Here's how the part is built. I have some questions about the finished solid (model axes, mm). A direction names the side the tool comes from. Give positions to 0.01 mm unless a question says otherwise; leave off trailing zeros. Write each loop counter-clockwise with the first axis right and the second up, starting at its lowest first coordinate (ties: lowest second). Pieces come first, ordered by that corner, then holes. Notation, with made-up numbers: M 78.25,42.5 L 128.25,42.5 A35 cw 128.25,79.5 Z; hole C 22,77 d1. An arc over 180 degrees is marked long. Use one line per item in the form item = value. Start each with the question number.
Autodesk Inventor part; units mm, degrees
ref_plane "YZ Plane" through (0, 0, 0) normal (1, 0, 0) x (0, 1, 0)
ref_plane "XZ Plane" through (0, 0, 0) normal (0, 1, 0) x (-1, 0, 0)
ref_plane "XY Plane" through (0, 0, 0) normal (0, 0, 1) x (1, 0, 0)
sketch "Sketch1" plane through (0, 0, 0) normal (0, 0, 1) x (1, 0, 0)
  line L0 (0, 0) -> (0, -635)
  line L1 (0, 0) -> (572.8366, -208.4955)
  line L2 (0, 0) -> (609.6, 0) construction
  line L3 (572.8366, -208.4955) -> (572.8366, -303.1009)
  line L4 (572.8366, -303.1009) -> (0, -94.6054)
  line L5 (0, 0) -> (-101.6, 0)
  line L6 (-101.6, 0) -> (-101.6, -635)
  line L7 (-101.6, -635) -> (0, -635)
  dimension "d0" = 635
  dimension "d1" = 609.6
  dimension "d2" = 20
  dimension "d3" = 88.9
  dimension "d4" = 101.6
extrude "Extrusion1" add sketch "Sketch1" along normal mid plane 304.8 contours L0 L7 L6 L5
extrude "Extrusion2" add sketch "Sketch1" along normal mid plane 44.45 contours L1 L3 L4 L0
properties part number "GarageSegment" material "Wood (Walnut)"
1) Suppose I cut it at B-B, the plane z = 42.5. List the corners of the cut face in (x, y) for me, and give its area (3 significant figures).
2) Suppose I cut it at A-A, the plane y = -245. List the corners of the cut face in (x, z) for me (3 decimals), and give its area (3 significant figures).
3) Suppose I cut it at C-C, the plane y = -527. List the corners of the cut face in (x, z) for me.
4) Thinking about a two-plate mould opening in X: for faces 3 (the face through (-101.6, -313, -2)), 4 (the face through (285, -140, 22.225)), 5 (the face through (290.428, -200.313, -0.311)), 6 (the face through (282.41, -102.79, -0.31)), which applies, released by +X, released by -X, zero draft, split by the parting line, or undercut?
5) Will these pins go through, and if not, where does the flat tip stop? P1, Ø12, axis at y = -402, z = 7.5, coming from the +X side; P2, Ø5, axis at x = 384.5, y = -154.5, coming from the -Z side (3 decimals); P3, Ø6, axis at x = 3.5, z = 110, coming from the +Y side; P4, Ø3, axis at x = 261.5, z = 20.5, coming from the -Y side.
6) On a 3-axis mill with a long thin cutter (end or side, diameter ignored), from which of +Z, -Z, +X, -X, +Y, -Y can I reach the whole of each face in a straight line? I mean faces 1 (the face through (-50, 0, -2)), 2 (the face through (285, -140, -22.225)). Say none if no direction works.
7) Please list where these lines run through material, in increasing order: line 1 (X direction, y = -586, z = 3.5); line 2 (Z direction, x = 428, y = -161) (3 decimals); line 3 (Y direction, x = 521.5, z = -10).
Checks:
q1.outline = M -101.6,-635 L 0,-635 L 0,0 L -101.6,0 Z
q1.area = 64,500 mm^2
q2.outline = M -101.6,-152.4 L 0,-152.4 L 0,152.4 L -101.6,152.4 Z; M 413.206,-22.225 L 572.837,-22.225 L 572.837,22.225 L 413.206,22.225 Z
q2.area = 38,100 mm^2
q3.outline = M -101.6,-152.4 L 0,-152.4 L 0,152.4 L -101.6,152.4 Z
q4.face_3 = released by -X
q4.face_4 = zero draft
q4.face_5 = undercut
q4.face_6 = released by +X
q5.P1 = 0
q5.P2 = -22.225
q5.P3 = through
q5.P4 = -190.33
q6.face_1 = +Z, -Z, +X, -X, +Y
q6.face_2 = -Z, +X, +Y, -Y
q7.line_1 = -101.6 to 0
q7.line_2 = -22.225 to 22.225
q7.line_3 = -284.42 to -189.81
